Read the model definition and answer for the solid it produces. Units are mm, in the model's axes. Coordinates: 2 decimals unless noted, no trailing zeros. Loops run counter-clockwise (first coordinate to the right, second up) from the corner with the lowest first, then second, coordinate; pieces in that order, holes last.
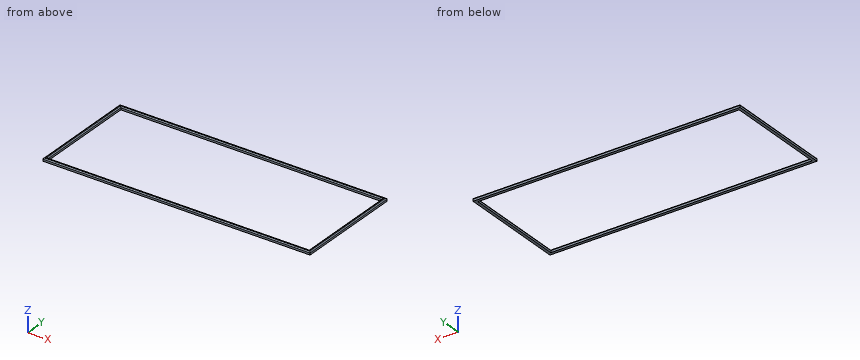
Autodesk Inventor part; units mm, degrees
ref_plane "YZ Plane" through (0, 0, 0) normal (1, 0, 0) x (0, 1, 0)
ref_plane "XZ Plane" through (0, 0, 0) normal (0, 1, 0) x (-1, 0, 0)
ref_plane "XY Plane" through (0, 0, 0) normal (0, 0, 1) x (1, 0, 0)
sketch "Skizze1" plane through (0, 0, 0) normal (0, 0, 1) x (1, 0, 0)
  line L0 (-55.6, 0) -> (333.6, 0)
  line L1 (0, -22.6) -> (0, 135.6)
  line L2 (3, 3) -> (275, 3)
  line L3 (275, 3) -> (275, 110)
  line L4 (275, 110) -> (3, 110)
  line L5 (3, 110) -> (3, 3)
  line L6 (0, 0) -> (278, 0)
  line L7 (278, 0) -> (278, 113)
  line L8 (278, 113) -> (0, 113)
  line L9 (0, 113) -> (0, 0)
  point P0 (0, 113)
  point P1 (278, 0)
  dimension "d0" = 272
  dimension "d1" = 107
  dimension "d2" = 3
  dimension "d3" = 3
  dimension "d4" = 3
  dimension "d5" = 3
extrude "Extrusion1" add sketch "Skizze1" along normal blind 3
fillet "Rundung1" radius 1 8 edges at (139, 110, 3) (139, 113, 3) (275, 56.5, 3) (278, 56.5, 3) (0, 56.5, 3) (3, 56.5, 3) (139, 3, 3) (139, 0, 3)
properties part number "Dichtung_1" material "Gummi"
Q1. A cutting plane is placed at A-A (x = 64). Give the vertices of the cut face in (y, z), then the cut area to 3 significant figures.
Findings below:
outline: (0, 0) - (3, 0) - (3, 2) arc R1 ccw to (2, 3) - (1, 3) arc R1 ccw to (0, 2) - close; (110, 0) - (113, 0) - (113, 2) arc R1 ccw to (112, 3) - (111, 3) arc R1 ccw to (110, 2) - close
area: 17.1 mm2
Q2. A cutting plane is placed at C-C (z = 1.35). Give the vertices of the cut face in (x, y), then the cut area to 3 significant figures.
Findings below:
outline: (0, 0) - (278, 0) - (278, 113) - (0, 113) - close; hole (3, 3) - (275, 3) - (275, 110) - (3, 110) - close
area: 2,310 mm2
Q3. Straight lines are drawn through the part: probe 1 along X at (y, z) = (5.5, 0.55); probe 2 along Y at (x, z) = (112, 0.4); probe 3 along Y at (x, z) = (79, 2.6). For each, find the intervals that lie inside material, in ascending order.
Findings below:
probe 1: x = 0 to 3, 275 to 278
probe 2: y = 0 to 3, 110 to 113
probe 3: y = 0.2 to 2.8, 110.2 to 112.8
Q4. A cutting plane is placed at B-B (y = 36). Give the vertices of the cut face in (x, z), then the cut area to 3 significant figures.
Findings below:
outline: (0, 0) - (3, 0) - (3, 2) arc R1 ccw to (2, 3) - (1, 3) arc R1 ccw to (0, 2) - close; (275, 0) - (278, 0) - (278, 2) arc R1 ccw to (277, 3) - (276, 3) arc R1 ccw to (275, 2) - close
area: 17.1 mm2
